from build123d import *

# Parameters (mm, degrees)
SKETCH_1_W          = 135
SKETCH_1_H          = 20
EXTRUDE_3_DEPTH     = 10
CUT_EXTRUDE_1_DEPTH = 62.5
FILLET_1_R          = 2
SKETCH_4_W          = 25.5
SKETCH_4_H          = 20
EXTRUDE_5_DEPTH     = 10
SKETCH_5_R          = 1.35
CUT_EXTRUDE_2_DEPTH = 96.650405122
SKETCH_6_W          = 25
SKETCH_6_H          = 5
CUT_EXTRUDE_3_DEPTH = 95.069123521


with BuildPart() as part:
    # 草图1 → 凸台-拉伸3 (new body)
    with BuildSketch(Plane(origin=(0, 0, 0), x_dir=(1, 0, 0), z_dir=(0, 1, 0))):
        Rectangle(SKETCH_1_W, SKETCH_1_H)
    extrude(amount=EXTRUDE_3_DEPTH)

    # 草图2 → 切除-拉伸1 (cut, symmetric)
    with BuildSketch(Plane(origin=(0, 0, 0), x_dir=(0, 0, -1), z_dir=(1, 0, 0))):
        Polygon((-6, 10), (-2, 3), (-2, 0), (2, 0), (2, 3), (6, 10), align=None)
    extrude(amount=CUT_EXTRUDE_1_DEPTH, both=True, mode=Mode.SUBTRACT)

    # 圆角1
    fillet_1_edges = [part.edges().sort_by_distance(p)[0] for p in [
        (62.5, 6.5, 4),
        (62.5, 6.5, -4),
        (-62.5, 6.5, -4),
        (-62.5, 6.5, 4),
        (-62.5, 1.5, -2),
        (62.5, 1.5, -2),
        (62.5, 1.5, 2),
        (-62.5, 1.5, 2),
    ]]
    fillet(fillet_1_edges, radius=FILLET_1_R - 0.0001)  # a hair under: the kernel refuses the full size

    # 草图4 → 凸台-拉伸5 (add)
    with BuildSketch(Plane(origin=(0, 10, 0), x_dir=(1, 0, 0), z_dir=(0, 1, 0))):
        with Locations((80.25, 0)):
            Rectangle(SKETCH_4_W, SKETCH_4_H)
    extrude(amount=-EXTRUDE_5_DEPTH)

    # 草图5 → 切除-拉伸2 (cut, through all)
    with BuildSketch(Plane(origin=(0, 0, -10), x_dir=(-1, 0, 0), z_dir=(0, 0, -1))):
        with Locations((-89, 5)):
            Circle(SKETCH_5_R)
        with Locations((-73, 5)):
            Circle(SKETCH_5_R)
    extrude(amount=-CUT_EXTRUDE_2_DEPTH, mode=Mode.SUBTRACT)

    # 草图6 → 切除-拉伸3 (cut, through all)
    with BuildSketch(Plane(origin=(0, 10, 0), x_dir=(1, 0, 0), z_dir=(0, 1, 0))):
        with Locations((80.5, -7.5)):
            Rectangle(SKETCH_6_W, SKETCH_6_H)
        with Locations((80.5, 7.5)):
            Rectangle(SKETCH_6_W, SKETCH_6_H)
    extrude(amount=-CUT_EXTRUDE_3_DEPTH, mode=Mode.SUBTRACT)


solid = part.part
Read the model definition and answer for the solid it produces. Units are mm, in the model's axes. A direction names the side the tool comes from. Coordinates: 2 decimals unless noted, no trailing zeros. Order: outer loops, then holes, each group sorted by start corner. A loop starts at its lowest first (then second) coordinate and runs counter-clockwise, first axis right, second up. Notation, with made-up numbers: M 9.25,51.5 L 33.25,51.5 A20 cw 33.25,90.5 Z; hole C 66,82 d9. An arc over 180 degrees is marked long. Put each result on its own line as item: value. Start each with the question number.
Item 1: Section A-A, the plane x = 89 is taken. Determine the outline of the cut face in (y, z).
Item 2: Section B-B, the plane z = -8.25 is taken. Determine the outline of the cut face in (x, y).
Item 3: The mould has two halves that part along X. Classify faces 5 (the face through (0.8, 6.5, 4)), 6 (the face through (71.753, 4.483, -0.07)), 7 (the face through (93, 5, 0)), 8 (the face through (11.6, 0, -2.4)): +X half, -X half, draft (parallel to the pull), parting line (faces both ways), or undercut.
Item 4: Given pin 1 Ø2.5 at (y, z) = (5.5, 6.5) entering from +X; pin 2 Ø5 at (x, y) = (86, 4) entering from -Z, each flat-ended and moving along its own axis, determine where each tip first touches the part or whether it passes through.
Item 5: Consider probe 1 along Z at (x, y) = (49.5, 2.5); probe 2 along Y at (x, z) = (89, -2); probe 3 along X at (y, z) = (1.25, -0.25). Determine where each line is inside the solid, lowest interval first. Write a range as [from, to].
Item 6: Section C-C, the plane y = 5 is taken. Count the separate pieces of the cut face and the enclosed holes in it, plus the area to 3 significant figures.
Item 7: For faces 1 (the face through (68, 5, -7)), 2 (the face through (62.5, 8, 0)), 3 (the face through (68, 5, 8)), 4 (the face through (1, 2, 2)), determine the directions among +Z, -Z, +X, -X, +Y, -Y from which every point of the face is accessible in a straight line to the end or side of a thin tool.
Item 8: Section D-D, the plane x = 9 is taken. Determine the outline of the cut face in (y, z).
Computed:
1. outline: M 0,-5 L 3.65,-5 L 3.65,5 L 0,5 Z; M 6.35,-5 L 10,-5 L 10,5 L 6.35,5 Z
2. outline: M -67.5,0 L 68,0 L 68,10 L -67.5,10 Z
3. face 5: undercut
3. face 6: undercut
3. face 7: +X half
3. face 8: draft
4. pin 1: stops at x = 68
4. pin 2: stops at z = -5
5. probe 1: z = [-10, -2], [2, 10]
5. probe 2: y = [0, 3.65], [6.35, 10]
5. probe 3: x = [-67.5, -62.48], [62.48, 93]
6. separate pieces: 3
6. enclosed holes: 1
6. area: 2,120 mm2
7. face 1: -Z, +X, +Y, -Y
7. face 2: +Y
7. face 3: +Z, +X, +Y, -Y
7. face 4: +Y, -Y
8. outline: M 0,-10 L 10,-10 L 10,-6 L 3,-2 L 0,-2 Z; M 0,2 L 3,2 L 10,6 L 10,10 L 0,10 Z
